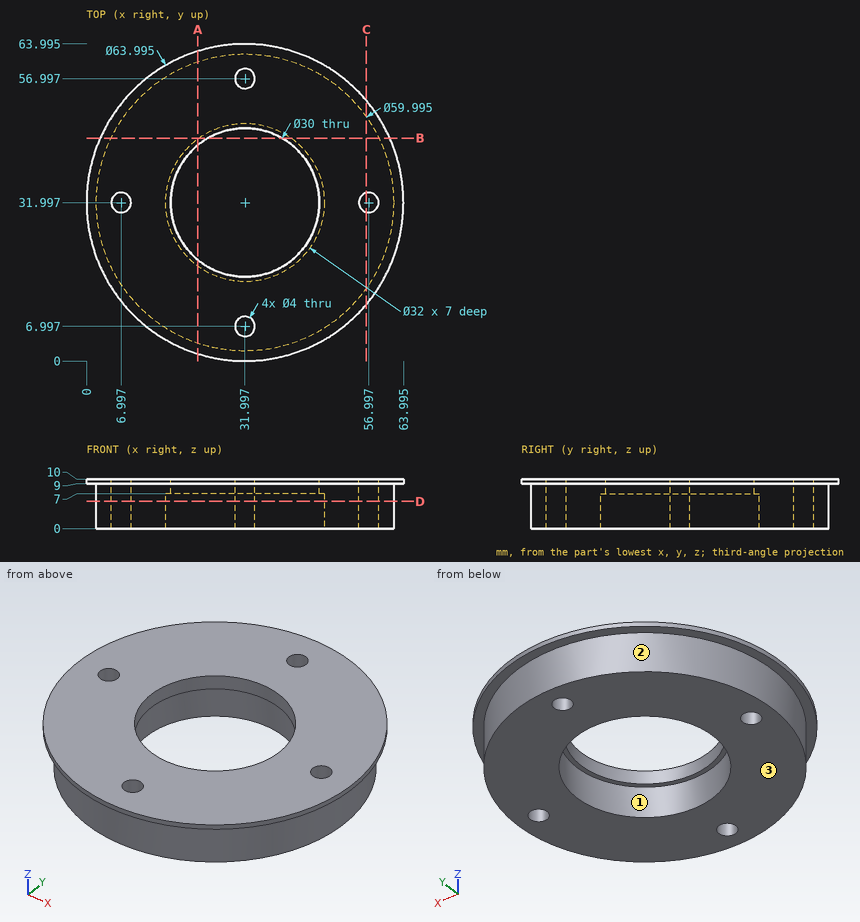
Print and shaded views of the part. All mm, measured from the part's lowest x, y and z. Coordinates: 2 decimals unless noted, no trailing zeros. Order: outer loops, then holes, each group sorted by start corner. A loop starts at its lowest first (then second) coordinate and runs counter-clockwise, first axis right, second up. Notation, with made-up numbers: M -28,71 L -6,71 A18 cw -6,96 Z; hole C 22,-28 d7. An arc over 180 degrees is marked long. Write each question's results on one line, items separated by ' | '. Start each with the question number.
Q1. Cut at C-C (x = 56.5). List the corners of the cut face in (y, z) (1 decimal).
Q2. Pull direction Y, two halves, no side cores. Call the marked faces 1, 2 and 3: +Y half, -Y half, draft (parallel to the pull), parting line (faces both ways), or undercut.
Q3. Cut at A-A (x = 22.5). List the corners of the cut face in (y, z), then the cut area to 3 significant figures.
Q4. Drill centre lines: probe 1 along Y at (x, z) = (32, 7.5) (1 decimal); probe 2 along X at (y, z) = (34.5, 2.75) (1 decimal); probe 3 along X at (y, z) = (41, 7.5) (1 decimal). Where is each one in solid material? Low to high. Write a range as from..to.
Q5. Cut at B-B (y = 45). List the corners of the cut face in (x, z) (1 decimal), then the cut area to 3 significant figures.
Q6. Cut at D-D (z = 5.5). List the corners of the cut face in (x, y) (1 decimal), then the cut area to 3 significant figures.
Q7. Flat gauge pins, fed straight in: P1, Ø2, axis at x = 41.5, z = 4.5, coming from the +Y side (1 decimal); P2, Ø3, axis at x = 57, y = 32, coming from the -Z side; P3, Ø6, axis at y = 7.5, z = 5.5, coming from the -X side (1 decimal); P4, Ø1.5, axis at x = 9, y = 9, coming from the -Z side. Where does each tip first touch, or does it go through?
Found:
1) outline: M 11.4,9 L 14.7,9 L 14.7,0 L 30.1,0 L 30.1,10 L 11.4,10 Z; M 33.9,0 L 49.3,0 L 49.3,9 L 52.6,9 L 52.6,10 L 33.9,10 Z
2) face 1: undercut | face 2: parting line | face 3: draft
3) outline: M 1.44,9 L 3.54,9 L 3.54,0 L 19.12,0 L 19.12,7 L 20.39,7 L 20.39,10 L 1.44,10 Z; M 43.61,7 L 44.87,7 L 44.87,0 L 60.45,0 L 60.45,9 L 62.55,9 L 62.55,10 L 43.61,10 Z | area: 323 mm²
4) probe 1: 2..5, 9..17, 47..55, 59..62 | probe 2: 2.1..16.2, 47.8..61.9 | probe 3: 3.4..20, 44..60.6
5) outline: M 2.8,9 L 5,9 L 5,0 L 22.7,0 L 22.7,7 L 24.5,7 L 24.5,10 L 2.8,10 Z; M 39.5,7 L 41.3,7 L 41.3,0 L 59,0 L 59,9 L 61.2,9 L 61.2,10 L 39.5,10 Z | area: 370 mm²
6) outline: C 32,32 d60; hole C 7,32 d4; hole C 32,32 d32; hole C 32,7 d4; hole C 32,57 d4; hole C 57,32 d4 | area: 1,970 mm²
7) P1: y = 60.8 | P2: through | P3: x = 11.1 | P4: z = 9
